from build123d import *

# Parameters (mm, degrees)
SKETCH_1_W           = 10.16
SKETCH_1_H           = 6.35
EXTRUDE_1_DEPTH      = 5.08
SKETCH_2_W           = 9.16
SKETCH_2_H           = 5.35
CUT_EXTRUDE_1_DEPTH  = 4.08
SKETCH_3_W           = 2
SKETCH_3_H           = 4.08
CUT_EXTRUDE_2_DEPTH  = 1
EXTRUDE_2_DEPTH      = 2
EXTRUDE_2_DEPTH_BACK = 3.58
SKETCH_4_W           = 0.75
SKETCH_4_H           = 0.75


with BuildPart() as part:
    # 草图1 → 拉伸1 (new body)
    with BuildSketch(Plane(origin=(0, 0, 0), x_dir=(1, 0, 0), z_dir=(0, 1, 0))):
        Rectangle(SKETCH_1_W, SKETCH_1_H)
    extrude(amount=EXTRUDE_1_DEPTH)

    # 草图2 → 切除-拉伸1 (cut)
    with BuildSketch(Plane(origin=(0, 5.08, 0), x_dir=(-1, 0, 0), z_dir=(0, 1, 0))):
        Rectangle(SKETCH_2_W, SKETCH_2_H)
    extrude(amount=-CUT_EXTRUDE_1_DEPTH, mode=Mode.SUBTRACT)

    # 草图3 → 切除-拉伸2 (cut)
    with BuildSketch(Plane.XY.offset(3.175)):
        with Locations((0, 3.04)):
            Rectangle(SKETCH_3_W, SKETCH_3_H)
    extrude(amount=-CUT_EXTRUDE_2_DEPTH, mode=Mode.SUBTRACT)

    # 草图4 → 拉伸2 (add, two sides: drawn at the far end of the back side and taken through both)
    with BuildSketch(Plane.XZ.offset(-EXTRUDE_2_DEPTH_BACK)):
        with Locations((0, 0.635)):
            Rectangle(SKETCH_4_W, SKETCH_4_H)
        with Locations((2.54, 0.635)):
            Rectangle(SKETCH_4_W, SKETCH_4_H)
        with Locations((-2.54, 0.635)):
            Rectangle(SKETCH_4_W, SKETCH_4_H)
    extrude(amount=EXTRUDE_2_DEPTH + EXTRUDE_2_DEPTH_BACK)


solid = part.part
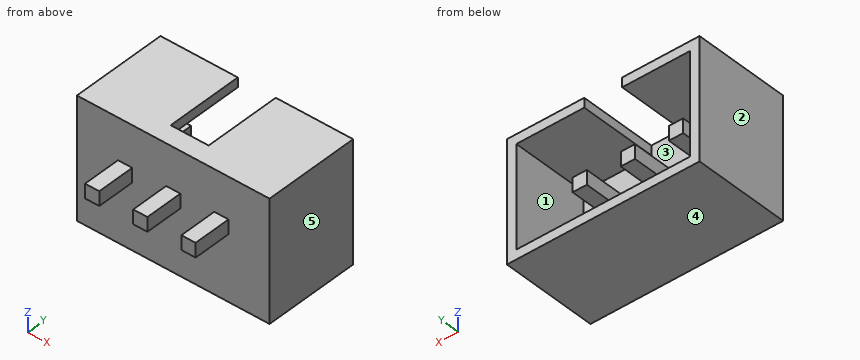
CAD build for the part. Positions are in the model's coordinates, mm. Face numbers are marked on the shaded views. A direction names the side the tool comes from. Coordinates: 2 decimals unless noted, no trailing zeros. Order: outer loops, then holes, each group sorted by start corner. A loop starts at its lowest first (then second) coordinate and runs counter-clockwise, first axis right, second up. Notation, with made-up numbers: (17, 47.25) -> (41, 47.25) arc R14 cw to (41, 68.25) -> close; hole circle Ø5 at (-13, -19.5). An arc over 180 degrees is marked (long way). Answer in a Markdown table with one row per item.
1) Which spindle directions (+Z, -Z, +X, -X, +Y, -Y) get a long thin tool onto all of the face, cutting with end or side? Do the marked faces 1 and 2. Say none if no direction does.
Check values:
| item | result |
|---|---|
| face 1 | +Y |
| face 2 | +Z, -Z, -X, +Y, -Y |
2) Drill centre lines: line 1 (Z direction, x = 2.75, y = 1.5) (3 decimals); line 2 (X direction, y = -0.25, z = 0.5) (3 decimals); line 3 (Z direction, x = 2.75, y = 4) (3 decimals). Where is each one in solid material? Low to high.
Check values:
| item | result |
|---|---|
| line 1 | -3.175 to -2.675, 0.26 to 1.01, 2.675 to 3.175 |
| line 2 | -2.915 to -2.165, -0.375 to 0.375, 2.165 to 2.915 |
| line 3 | -3.175 to -2.675, 2.675 to 3.175 |
3) Band-saw the part on C-C (y = 2). List the corners of the cut face in (x, z) (3 decimals), and give its area (3 significant figures).
Check values:
| item | result |
|---|---|
| outline | (-5.08, -3.175) -> (5.08, -3.175) -> (5.08, 3.175) -> (1, 3.175) -> (1, 2.675) -> (4.58, 2.675) -> (4.58, -2.675) -> (-4.58, -2.675) -> (-4.58, 2.675) -> (-1, 2.675) -> (-1, 3.175) -> (-5.08, 3.175) -> close; (-2.915, 0.26) -> (-2.165, 0.26) -> (-2.165, 1.01) -> (-2.915, 1.01) -> close; (-0.375, 0.26) -> (0.375, 0.26) -> (0.375, 1.01) -> (-0.375, 1.01) -> close; (2.165, 0.26) -> (2.915, 0.26) -> (2.915, 1.01) -> (2.165, 1.01) -> close |
| area | 16.2 mm2 |
4) Mould opens along X. For the marked faces 3, 4 and 5 say: pulls with the +X half, pulls with the -X half, needs draft (parallel to the pull), parting line crosses it, or undercut.
Check values:
| item | result |
|---|---|
| face 3 | undercut |
| face 4 | needs draft |
| face 5 | pulls with the +X half |
5) Band-saw the part on D-D (x = -0.25). List the corners of the cut face in (y, z) (3 decimals), and give its area (3 significant figures).
Check values:
| item | result |
|---|---|
| outline | (-2, 0.26) -> (0, 0.26) -> (0, -3.175) -> (5.08, -3.175) -> (5.08, -2.675) -> (1, -2.675) -> (1, 0.26) -> (3.58, 0.26) -> (3.58, 1.01) -> (1, 1.01) -> (1, 3.175) -> (0, 3.175) -> (0, 1.01) -> (-2, 1.01) -> close |
| area | 11.8 mm2 |
6) Band-saw the part on A-A (y = -1.5). List the corners of the cut face in (x, z) (3 decimals), and give its area (3 significant figures).
Check values:
| item | result |
|---|---|
| outline | (-2.915, 0.26) -> (-2.165, 0.26) -> (-2.165, 1.01) -> (-2.915, 1.01) -> close; (-0.375, 0.26) -> (0.375, 0.26) -> (0.375, 1.01) -> (-0.375, 1.01) -> close; (2.165, 0.26) -> (2.915, 0.26) -> (2.915, 1.01) -> (2.165, 1.01) -> close |
| area | 1.69 mm2 |
7) Band-saw the part on B-B (z = -1.5). List the corners of the cut face in (x, y).
Check values:
| item | result |
|---|---|
| outline | (-5.08, 0) -> (5.08, 0) -> (5.08, 5.08) -> (4.58, 5.08) -> (4.58, 1) -> (-4.58, 1) -> (-4.58, 5.08) -> (-5.08, 5.08) -> close |
8) Flat gauge pins, fed straight in: P1, Ø0.6, axis at y = -1.5, z = 0.5, coming from the -X side (3 decimals); P2, Ø0.8, axis at y = -1.5, z = 1, coming from the +X side (3 decimals); P3, Ø2, axis at x = 3, z = 2.5, coming from the -Y side. Where does each tip first touch, or does it go through?
Check values:
| item | result |
|---|---|
| P1 | x = -2.915 |
| P2 | x = 2.915 |
| P3 | y = 0 |
